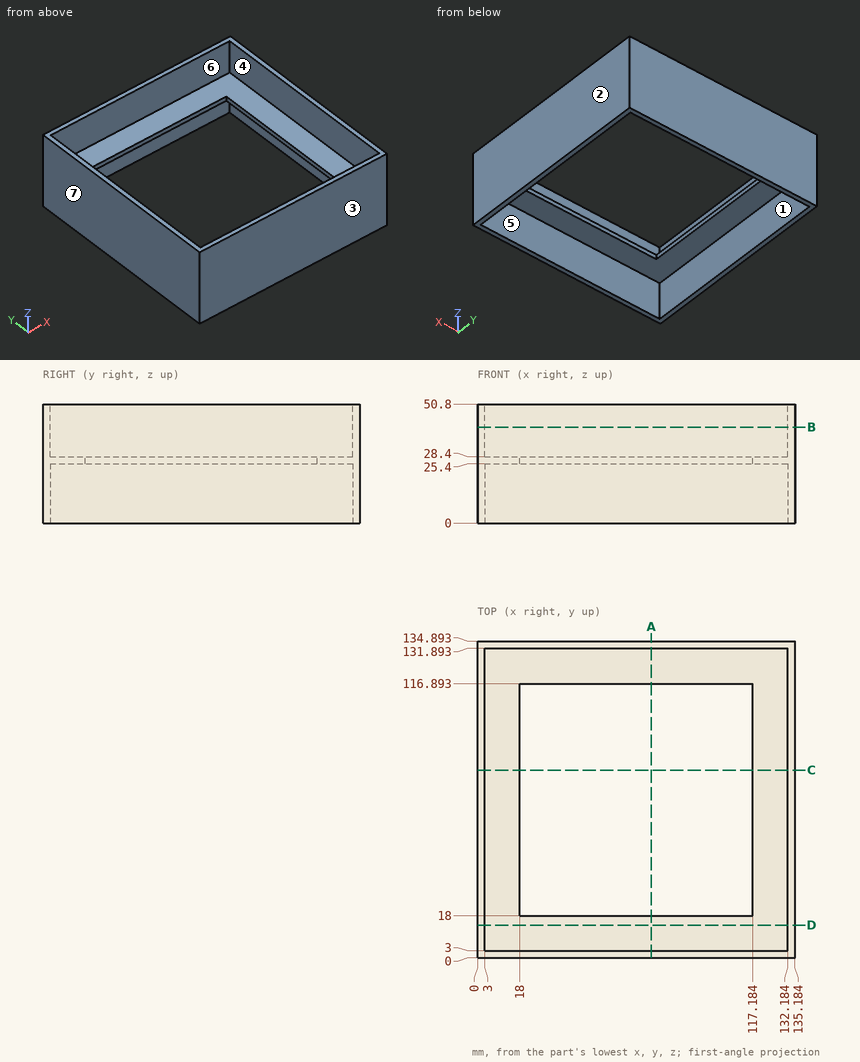
Answer from the drawing. Dimensions are ordinates in mm from the lowest x, y and z of the part. A direction names the side the tool comes from. Give positions to 0.01 mm unless a question says otherwise; leave off trailing zeros. Write each loop counter-clockwise with the first axis right and the second up, starting at its lowest first coordinate (ties: lowest second). Pieces come first, ordered by that corner, then holes.
1) Find the intervals of material crossed by L1, parallel to X at y = 28, z = 46 (1 decimal); L2, parallel to Y at x = 12, z = 38.5; L3, parallel to Z at x = 73.5, y = 7, in increasing order.
2) Section C-C (y = 80) is taken. Write down the section's boundary in (x, z) (1 decimal).
3) Section B-B (z = 41) is taken. Write down the section's boundary in (x, y) (1 decimal).
4) Section A-A (x = 74) is taken. Write down the section's boundary in (y, z), and give its area (3 significant figures).
5) Given P1, Ø12, axis at x = 32.5, y = 23.5, coming from the +Z side; P2, Ø8, axis at x = 113, y = 53, coming from the +Z side, each flat-ended and moving along its own axis, determine where each tip first touches the part or whether it passes through.
6) For a pull along Y with two mould halves and no side action, classify the marked faces 1, 2, 3 and 4 as pulls with the +Y half, pulls with the -Y half, needs draft (parallel to the pull), parting line crosses it, or undercut.
7) Section D-D (y = 14) is taken. Write down the section's boundary in (x, z) (1 decimal).
8) A tool of negligible diameter and unlimited length cuts with its end or side. For the marked faces 5, 6 and 7, from which of +Z, -Z, +X, -X, +Y, -Y can it reach the whole face along a straight path? Write none if from no direction.
Response:
1. L1: x = 0 to 3, 132.2 to 135.2
1. L2: y = 0 to 3, 131.89 to 134.89
1. L3: z = 25.4 to 28.4
2. outline: (0, 0) - (3, 0) - (3, 25.4) - (18, 25.4) - (18, 28.4) - (3, 28.4) - (3, 50.8) - (0, 50.8) - close; (117.2, 25.4) - (132.2, 25.4) - (132.2, 0) - (135.2, 0) - (135.2, 50.8) - (132.2, 50.8) - (132.2, 28.4) - (117.2, 28.4) - close
3. outline: (0, 0) - (135.2, 0) - (135.2, 134.9) - (0, 134.9) - close; hole (3, 3) - (132.2, 3) - (132.2, 131.9) - (3, 131.9) - close
4. outline: (0, 0) - (3, 0) - (3, 25.4) - (18, 25.4) - (18, 28.4) - (3, 28.4) - (3, 50.8) - (0, 50.8) - close; (116.89, 25.4) - (131.89, 25.4) - (131.89, 0) - (134.89, 0) - (134.89, 50.8) - (131.89, 50.8) - (131.89, 28.4) - (116.89, 28.4) - close
4. area: 395 mm2
5. P1: stops at z = 28.4
5. P2: passes through
6. face 1: undercut
6. face 2: needs draft
6. face 3: pulls with the -Y half
6. face 4: undercut
7. outline: (0, 0) - (3, 0) - (3, 25.4) - (132.2, 25.4) - (132.2, 0) - (135.2, 0) - (135.2, 50.8) - (132.2, 50.8) - (132.2, 28.4) - (3, 28.4) - (3, 50.8) - (0, 50.8) - close
8. face 5: -Z
8. face 6: +Z
8. face 7: +Z, -Z, -X, +Y, -Y
